Autodesk Inventor part; units mm, degrees
ref_plane "YZ Plane" through (0, 0, 0) normal (1, 0, 0) x (0, 1, 0)
ref_plane "XZ Plane" through (0, 0, 0) normal (0, 1, 0) x (-1, 0, 0)
ref_plane "XY Plane" through (0, 0, 0) normal (0, 0, 1) x (1, 0, 0)
sketch "Boceto1" plane through (0, 0, 0) normal (0, 1, 0) x (-1, 0, 0)
  line L0 (0, 0) -> (11.8, 0)
  line L1 (11.8, 0) -> (11.8, -23.2)
  line L2 (11.8, -23.2) -> (0, -23.2)
  line L3 (0, -23.2) -> (0, 0)
  dimension "d0" = 11.8
  dimension "d1" = 23.2
extrude "Extrusión1" add sketch "Boceto1" along normal blind 23
sketch "Boceto2" plane through (0, 0, 0) normal (1, 0, 0) x (0, 0, -1)
  line L0 (0, 0) -> (0, 23)
  line L1 (0, 0) -> (0, 16.4)
  line L2 (0, 16.4) -> (-4.7, 16.4)
  line L3 (-4.7, 16.4) -> (-4.7, 18.8)
  line L4 (-4.7, 18.8) -> (0, 18.8)
  line L5 (23.2, 0) -> (23.2, 23)
  line L6 (23.2, 16.4) -> (27.9, 16.4)
  line L7 (27.9, 16.4) -> (27.9, 18.8)
  line L8 (27.9, 18.8) -> (23.2, 18.8)
  line L9 (0, 18.8) -> (0, 16.4)
  line L10 (23.2, 18.8) -> (23.2, 16.4)
  dimension "d4" = 16.4
  dimension "d5" = 4.7
  dimension "d6" = 2.4
  dimension "d7" = 4.7
extrude "Extrusión2" add sketch "Boceto2" against normal blind 11.8
move faces "Desplazar1" translate (0.7, 0, 0) faces at (0, 5.4667, -15.4667)
sketch "Boceto4" plane through (-11.8, 18.8, 4.7) normal (0, 1, 0) x (1, 0, 0)
  line L0 (12.5, 0) -> (12.5, 4.7)
  line L1 (0, 0) -> (12.5, 0)
  line L2 (12.5, 0) -> (0, 0)
  line L3 (6.25, 0) -> (6.25, 1.9)
  line L4 (0, 32.6) -> (0, 27.9)
  line L5 (12.5, 32.6) -> (0, 32.6)
  line L6 (0, 32.6) -> (12.5, 32.6)
  line L7 (6.25, 32.6) -> (6.25, 30.7)
  circle A0 centre (6.25, 1.9) radius 1
  circle A1 centre (6.25, 30.7) radius 1
  point P0 (11.8, 4.7)
  dimension "d13" = 1.9
  dimension "d14" = 1.9
  dimension "d15" = 2
  dimension "d16" = 2
extrude "Extrusión3" cut sketch "Boceto4" against normal blind 2.4
sketch "Boceto5" plane through (0, 23, 0) normal (0, 1, 0) x (1, 0, 0)
  line L0 (-11.8, 23.2) -> (-11.8, 0)
  line L1 (-11.8, 0) -> (0.7, 0)
  line L2 (-11.8, 0) -> (0.7, 0)
  line L3 (0.7, 0) -> (0.7, 15)
  line L4 (0.7, 0) -> (0.7, 23.2)
  line L5 (0.7, 15) -> (-11.8, 15)
  line L6 (-11.8, 15) -> (-11.8, 0)
  point P0 (0, 0)
  dimension "d19" = 15
extrude "Extrusión4" add sketch "Boceto5" along normal blind 4.3
sketch "Boceto6" plane through (0, 27.3, 0) normal (0, 1, 0) x (1, 0, 0)
  line L0 (-11.8, 0) -> (0.7, 0)
  line L1 (-5.55, 0) -> (-5.55, 5)
  circle A0 centre (-5.55, 5) radius 2.4
  point P0 (0, 0)
  dimension "d22" = 5
  dimension "d23" = 4.8
extrude "Extrusión5" add sketch "Boceto6" along normal blind 5
sketch "Boceto7" plane through (0, 27.3, 0) normal (0, 1, 0) x (1, 0, 0)
  line L0 (-11.8, 0) -> (0.7, 0)
  line L1 (-5.55, 0) -> (-5.55, 6.25)
  arc A0 (-7.9995, 12) -> (-3.1005, 12) centre (-5.55, 6.25) ccw
  line L2 (0.7, 15) -> (-11.8, 15)
  arc A1 (-3.1005, 12) -> (-7.9995, 12) centre (-5.55, 12.5) ccw
  line L3 (0.7, 0) -> (-11.8, 0)
  line L4 (-11.8, 15) -> (-11.8, 0)
  line L5 (-11.8, 0) -> (-11.8, 15)
  line L6 (-11.8, 15) -> (0.7, 15)
  line L7 (0.7, 23.2) -> (0.7, 0)
  line L8 (0.7, 0) -> (0.7, 15)
  point P0 (0, 0)
  dimension "d26" = 6.25
extrude "Extrusión6" cut sketch "Boceto7" against normal blind 4.3 contours L4 A0 L0 | A0 L7 L0 | L4 L2 A1 A0 | A0 A1 L2 L7
sketch "Boceto9" plane through (-11.8, 0, 0) normal (0, 0, 1) x (1, 0, 0)
  line L0 (12.5, 0) -> (0, 0)
  line L1 (12.5, 0) -> (6.25, 0)
  line L2 (6.25, 0) -> (6.25, 3)
  line L3 (8.75, 3) -> (3.75, 3)
  line L4 (6.25, 3) -> (8.75, 3)
  line L5 (8.75, 0) -> (8.75, 3)
  line L6 (8.75, 3) -> (8.75, 0)
  line L7 (6.25, 3) -> (3.75, 3)
  line L8 (3.75, 3) -> (3.75, 0)
  line L9 (3.75, 3) -> (3.75, 0)
  line L10 (3.75, 0) -> (6.25, 0)
  point P0 (11.8, 0)
  dimension "d35" = 3
  dimension "d36" = 2.5
extrude "Extrusión8" cut sketch "Boceto9" against normal blind 5
properties part number "microservo_FT"
CAD build for the part. Positions are in the model's coordinates, mm. A direction names the side the tool comes from. Give positions to 0.01 mm unless a question says otherwise; leave off trailing zeros. Loops run counter-clockwise (first coordinate to the right, second up) from the corner with the lowest first, then second, coordinate; pieces in that order, holes last. Notation, with made-up numbers: M 29,56 L 79,56 A35 cw 79,92 Z; hole C -33.75,72.5 d4. An arc over 180 degrees is marked long. One line per question, with ' | ' between items. Start each with the question number.
1. 3-axis set-ups, long thin cutter, end or side, ignore diameter. For faces 1 (the face through (-5.79, 25.18, -0.005)), 2 (the face through (-1, 23, -1)), 3 (the face through (-6, 2, -5)), 4 (the face through (-5, 16.4, -24)): which of +Z, -Z, +X, -X, +Y, -Y reach the whole face in a straight line?
2. Saw through at C-C on y = 9. Give the cut face in (x, z), plus the area to 3 significant figures.
3. Probe L1, parallel to Z at x = -5.55, y = 16.95; L2, parallel to X at y = 17.8, z = 2.8; L3, parallel to Y at x = -6.25, z = 0.5. List the from-to ranges inside material, lowest first. Write a range as from..to.
4. Two-plate mould, pull along X, no slides. Class faces 5 (the face through (-5.09, 17.62, -25.11)), 6 (the face through (-6, 3, -2)), 7 (the face through (-5, 18, 4.7)), 8 (the face through (-11.8, 11, -12)): pulls with the +X half, pulls with the -X half, needs draft (parallel to the pull), parting line crosses it, or undercut.
5. Saw through at B-B on z = -12.5. Give the cut face in (x, y).
6. Flat gauge pins, fed straight in: pin 1 (2.5 mm diameter, centred on x = -5.55, z = 2.8, fed in from +Y); pin 2 (1.5 mm diameter, centred on x = -5, z = -2, fed in from -Y); pin 3 (2.5 mm diameter, centred on x = -5, z = -26, fed in from -Y); pin 4 (1.2 mm diameter, centred on x = -5.55, z = -26, fed in from +Y). Where does each tip first touch, or does it go through?
7. Saw through at D-D on z = -22.5. Give the cut face in (x, y), plus the area to 4 significant figures.
8. Saw through at A-A on z = 2.8. Give the cut face in (x, y), plus the area to 3 significant figures.
Result sheet:
1) face 1: +Y | face 2: +Z, +X, +Y | face 3: +Z, -Y | face 4: -Z, +X, -X, -Y
2) outline: M -11.8,-23.2 L 0.7,-23.2 L 0.7,0 L -11.8,0 Z | area: 290 mm^2
3) L1: z = -27.9..-27, -25..1.8, 3.8..4.7 | L2: x = -11.8..-6.55, -4.55..0.7 | L3: y = 16.4..18.8
4) face 5: undercut | face 6: undercut | face 7: needs draft | face 8: pulls with the -X half
5) outline: M -11.8,0 L 0.7,0 L 0.7,23 L -3.05,23 L -3.05,27.3 L -8.05,27.3 L -8.05,23 L -11.8,23 Z
6) pin 1: stops at y = 18.8 | pin 2: stops at y = 3 | pin 3: stops at y = 16.4 | pin 4: passes through
7) outline: M -11.8,0 L 0.7,0 L 0.7,23 L -11.8,23 Z | area: 287.5 mm^2
8) outline: M -11.8,16.4 L -6.55,16.4 L -6.55,18.8 L -11.8,18.8 Z; M -4.55,16.4 L 0.7,16.4 L 0.7,18.8 L -4.55,18.8 Z | area: 25.2 mm^2
